from build123d import *

# Parameters (mm, degrees)
EXTRUDE_1_DEPTH     = 88.9
SKETCH_4_R          = 1.5
SKETCH_4_W          = 31.75
SKETCH_4_H          = 3
SKETCH_4_W_2        = 3
SKETCH_4_H_2        = 31.75
CUT_EXTRUDE_1_DEPTH = 3
SKETCH_5_R          = 1.56
CUT_EXTRUDE_2_DEPTH = 3
SKETCH_7_R          = 4.635
SKETCH_7_R_2        = 2.23
CUT_EXTRUDE_3_DEPTH = 3
SKETCH_8_W          = 9.6
SKETCH_8_H          = 2.88
SKETCH_8_W_2        = 2.88
SKETCH_8_H_2        = 9.6
CUT_EXTRUDE_4_DEPTH = 3
SKETCH_9_R          = 3.175
CUT_EXTRUDE_5_DEPTH = 3
SKETCH_13_W         = 6.4135
SKETCH_13_H         = 6.4135
CUT_EXTRUDE_7_DEPTH = 5.08
FILLET_2_R          = 2.032
SKETCH_18_R         = 1.190625
SKETCH_18_W         = 19.446875
SKETCH_18_H         = 26.7890625
CUT_EXTRUDE_8_DEPTH = 3
SKETCH_19_W         = 2.804
SKETCH_19_H         = 10.5
CUT_EXTRUDE_9_DEPTH = 2000


with BuildPart() as part:
    # 스케치2 → 보스-돌출1 (new body)
    with BuildSketch(Plane.XY):
        Polygon((-44.45, 1.5), (44.45, 1.5), (83.82, 1.5), (83.82, -1.5), (44.45, -1.5), (-44.45, -1.5), align=None)
    extrude(amount=EXTRUDE_1_DEPTH)

    # 스케치4 → 컷-돌출1 (cut)
    with BuildSketch(Plane(origin=(0, 1.5, 0), x_dir=(1, 0, 0), z_dir=(0, 1, 0))):
        with Locations(Location((-41.275, -85.725, 0), (0, 0, 270))):
            Circle(SKETCH_4_R)
        with Locations(Location((-41.275, -3.175, 0), (0, 0, 270))):
            Circle(SKETCH_4_R)
        with Locations(Location((41.275, -3.175, 0), (0, 0, 270))):
            Circle(SKETCH_4_R)
        with Locations(Location((41.275, -85.725, 0), (0, 0, 270))):
            Circle(SKETCH_4_R)
        with Locations((0, -81.05)):
            Rectangle(SKETCH_4_W, SKETCH_4_H)
        with Locations((-36.6, -44.45)):
            Rectangle(SKETCH_4_W_2, SKETCH_4_H_2)
        with Locations((0, -7.85)):
            Rectangle(SKETCH_4_W, SKETCH_4_H)
        with Locations((36.6, -44.45)):
            Rectangle(SKETCH_4_W_2, SKETCH_4_H_2)
    extrude(amount=-CUT_EXTRUDE_1_DEPTH, mode=Mode.SUBTRACT)

    # 스케치5 → 컷-돌출2 (cut)
    with BuildSketch(Plane(origin=(0, 1.5, 0), x_dir=(1, 0, 0), z_dir=(0, 1, 0))):
        with Locations(Location((-14.431818182, -30.018181818, 0), (0, 0, 270))):
            Circle(SKETCH_5_R)
        with Locations(Location((14.431818182, -30.018181818, 0), (0, 0, 270))):
            Circle(SKETCH_5_R)
        with Locations(Location((14.431818182, -58.881818182, 0), (0, 0, 270))):
            Circle(SKETCH_5_R)
        with Locations(Location((-14.431818182, -58.881818182, 0), (0, 0, 270))):
            Circle(SKETCH_5_R)
    extrude(amount=-CUT_EXTRUDE_2_DEPTH, mode=Mode.SUBTRACT)

    # 스케치7 → 컷-돌출3 (cut)
    with BuildSketch(Plane(origin=(0, 1.5, 0), x_dir=(1, 0, 0), z_dir=(0, 1, 0))):
        with Locations(Location((14.431818182, -30.018181818, 0), (0, 0, 270))):
            Circle(SKETCH_7_R)
        with Locations((6.401818182, -47.508181818)):
            Circle(SKETCH_7_R_2)
        with Locations((6.401818182, -12.528181818)):
            Circle(SKETCH_7_R_2)
    extrude(amount=-CUT_EXTRUDE_3_DEPTH, mode=Mode.SUBTRACT)

    # 스케치8 → 컷-돌출4 (cut)
    with BuildSketch(Plane(origin=(0, 1.5, 0), x_dir=(1, 0, 0), z_dir=(0, 1, 0))):
        with Locations((-25.4, -7.85)):
            Rectangle(SKETCH_8_W, SKETCH_8_H)
        with Locations((-36.6, -19.05)):
            Rectangle(SKETCH_8_W_2, SKETCH_8_H_2)
        with Locations((36.6, -19.05)):
            Rectangle(SKETCH_8_W_2, SKETCH_8_H_2)
        with Locations((25.4, -7.85)):
            Rectangle(SKETCH_8_W, SKETCH_8_H)
        with Locations((36.6, -69.85)):
            Rectangle(SKETCH_8_W_2, SKETCH_8_H_2)
        with Locations((25.4, -81.05)):
            Rectangle(SKETCH_8_W, SKETCH_8_H)
        with Locations((-25.4, -81.05)):
            Rectangle(SKETCH_8_W, SKETCH_8_H)
        with Locations((-36.6, -69.85)):
            Rectangle(SKETCH_8_W_2, SKETCH_8_H_2)
    extrude(amount=-CUT_EXTRUDE_4_DEPTH, mode=Mode.SUBTRACT)

    # 스케치9 → 컷-돌출5 (cut)
    with BuildSketch(Plane(origin=(0, 1.5, 0), x_dir=(1, 0, 0), z_dir=(0, 1, 0))):
        with Locations(Location((0, -44.45, 0), (0, 0, 270))):
            Circle(SKETCH_9_R)
    extrude(amount=-CUT_EXTRUDE_5_DEPTH, mode=Mode.SUBTRACT)

    # 스케치13 → 컷-돌출7 (cut)
    with BuildSketch(Plane(origin=(0, 1.5, 0), x_dir=(1, 0, 0), z_dir=(0, 1, 0))):
        with Locations((-41.24325, -85.69325)):
            Rectangle(SKETCH_13_W, SKETCH_13_H)
        with Locations((-41.24325, -3.20675)):
            Rectangle(SKETCH_13_W, SKETCH_13_H)
        with Locations((41.24325, -3.20675)):
            Rectangle(SKETCH_13_W, SKETCH_13_H)
        with Locations((41.24325, -85.69325)):
            Rectangle(SKETCH_13_W, SKETCH_13_H)
    extrude(amount=-CUT_EXTRUDE_7_DEPTH, mode=Mode.SUBTRACT)

    # 필렛2
    fillet_2_edges = [part.edges().sort_by_distance(p)[0] for p in [
        (44.45, 0, 82.4865),
        (38.0365, 0, 82.4865),
        (44.45, 0, 6.4135),
        (38.0365, 0, 6.4135),
        (-38.0365, 0, 6.4135),
        (-38.0365, 0, 82.4865),
    ]]
    fillet(fillet_2_edges, radius=FILLET_2_R)

    # 스케치18 → 컷-돌출8 (cut)
    with BuildSketch(Plane(origin=(0, 1.5, 0), x_dir=(1, 0, 0), z_dir=(0, 1, 0))):
        with Locations(Location((50.95875, -56.1578125, 0), (0, 0, 180))):
            Circle(SKETCH_18_R)
        with Locations(Location((50.95875, -32.7421875, 0), (0, 0, 180))):
            Circle(SKETCH_18_R)
        with Locations((74.77125, -32.7421875)):
            Circle(SKETCH_18_R)
        with Locations((74.77125, -56.1578125)):
            Circle(SKETCH_18_R)
        with Locations((62.865, -44.45)):
            Rectangle(SKETCH_18_W, SKETCH_18_H)
    extrude(amount=-CUT_EXTRUDE_8_DEPTH, mode=Mode.SUBTRACT)

    # 스케치19 → 컷-돌출9 (cut)
    with BuildSketch(Plane(origin=(0, 1.5, 0), x_dir=(1, 0, 0), z_dir=(0, 1, 0))):
        with Locations((50.122375, -44.45)):
            Rectangle(SKETCH_19_W, SKETCH_19_H)
    extrude(amount=-CUT_EXTRUDE_9_DEPTH, mode=Mode.SUBTRACT)


solid = part.part
Verification items for the finished model (mm, model axes). A direction names the side the tool comes from. Give positions to 0.01 mm unless a question says otherwise; leave off trailing zeros. Write each loop counter-clockwise with the first axis right and the second up, starting at its lowest first coordinate (ties: lowest second). Pieces come first, ordered by that corner, then holes. Notation, with made-up numbers: M 6,45 L 44,45 A12 cw 44,58 Z; hole C -2,35.5 d3. An arc over 180 degrees is marked long. Put each result on its own line as item: value. Start each with the question number.
1. Section check A-A (x = 61). Record the cut outline in (y, z).
2. Section check C-C (x = -23). Record the cut outline in (y, z), and give its area (3 significant figures).
3. Scan lines: line 1 along X through (y, z) = (0.2, 66.5); line 2 along Z through (x, y) = (-14.5, 0.3); line 3 along Z through (x, y) = (-21, 0.95). Record each from-to range of solid material in increasing order. Write a range as [from, to].
4. Draft check along Z on faces 1 (the face through (-38.037, 0, 2)), 2 (the face through (41, 0, 82.486)), 3 (the face through (50, 0, 49.7)). Enter one of: +Z half, -Z half, draft (parallel to the pull), parting line (faces both ways), or undercut.
5. Set-up check for faces 4 (the face through (83.82, 0, 44)), 5 (the face through (35.1, 0, 45)), 6 (the face through (-42, 0, 82.486)): record each of +Z, -Z, +X, -X, +Y, -Y from which the full face is reachable in a straight line by a thin tool's end or side.
6. Go/stop test with flat-tipped pins: pin 1 Ø5 at (x, z) = (6.4, 12.53) entering from +Y; pin 2 Ø0.9 at (x, y) = (-41, 0.5) entering from +Z. Record where each tip stops, or that it passes through.
7. Section check D-D (x = 0). Record the cut outline in (y, z) (3 decimals), and give its area (3 significant figures).
8. Section check B-B (z = 22.5). Record the cut outline in (x, y).
Answer list:
1. outline: M -1.5,0 L 1.5,0 L 1.5,31.06 L -1.5,31.06 Z; M -1.5,57.84 L 1.5,57.84 L 1.5,88.9 L -1.5,88.9 Z
2. outline: M -1.5,0 L 1.5,0 L 1.5,6.41 L -1.5,6.41 Z; M -1.5,9.29 L 1.5,9.29 L 1.5,79.61 L -1.5,79.61 Z; M -1.5,82.49 L 1.5,82.49 L 1.5,88.9 L -1.5,88.9 Z
2. area: 249 mm2
3. line 1: [-44.45, -38.04], [-35.16, 35.16], [38.04, 83.82]
3. line 2: [0, 6.35], [9.35, 28.46], [31.58, 57.32], [60.44, 79.55], [82.55, 88.9]
3. line 3: [0, 6.41], [9.29, 79.61], [82.49, 88.9]
4. face 1: draft
4. face 2: +Z half
4. face 3: undercut
5. face 4: +Z, -Z, +X, +Y, -Y
5. face 5: +Y, -Y
5. face 6: +Z, -X, +Y, -Y
6. pin 1: y = 1.5
6. pin 2: z = 82.49
7. outline: M -1.5,0 L 1.5,0 L 1.5,6.35 L -1.5,6.35 Z; M -1.5,9.35 L 1.5,9.35 L 1.5,41.275 L -1.5,41.275 Z; M -1.5,47.625 L 1.5,47.625 L 1.5,79.55 L -1.5,79.55 Z; M -1.5,82.55 L 1.5,82.55 L 1.5,88.9 L -1.5,88.9 Z
7. area: 230 mm2
8. outline: M -44.45,-1.5 L -38.04,-1.5 L -38.04,1.5 L -44.45,1.5 Z; M -35.16,-1.5 L 35.16,-1.5 L 35.16,1.5 L -35.16,1.5 Z; M 38.04,-1.5 L 83.82,-1.5 L 83.82,1.5 L 38.04,1.5 Z
